from build123d import *

# Parameters (mm, degrees)
BOSS_EXTRUDE1_DEPTH  = 2
SKETCH2_W            = 8
SKETCH2_H            = 8
BOSS_EXTRUDE2_DEPTH  = 2
SKETCH3_W            = 8
SKETCH3_H            = 8
BOSS_EXTRUDE3_DEPTH  = 8
SKETCH4_R            = 3.5
CUT_EXTRUDE1_DEPTH   = 10
CUT_EXTRUDE2_REACH   = 4
SKETCH5_R            = 0.65
CUT_EXTRUDE3_REACH   = 3
SKETCH6_R            = 0.65
SKETCH10_R           = 0.65
BOSS_EXTRUDE6_DEPTH  = 3
SKETCH11_W           = 8
SKETCH11_H           = 2
BOSS_EXTRUDE7_DEPTH  = 8
SKETCH12_R           = 1
CUT_EXTRUDE5_DEPTH   = 8
SKETCH13_W           = 8
SKETCH13_H           = 12
BOSS_EXTRUDE8_DEPTH  = 2
SKETCH14_W           = 8
SKETCH14_H           = 4
BOSS_EXTRUDE9_DEPTH  = 1
BOSS_EXTRUDE10_DEPTH = 2
SKETCH18_R           = 0.65
BOSS_EXTRUDE11_DEPTH = 4
CUT_EXTRUDE6_REACH   = 6
SKETCH19_R           = 0.65
CUT_EXTRUDE7_REACH   = 4
SKETCH20_R           = 1.75


with BuildPart() as part:
    # Sketch1 → Boss-Extrude1 (new body)
    with BuildSketch(Plane(origin=(0, 0, 0), x_dir=(1, 0, 0), z_dir=(0, 1, 0))):
        Polygon((-16, 0), (0, 0), (0, 1), (-8, 1), (-8, 8), (-16, 8), align=None)
    extrude(amount=BOSS_EXTRUDE1_DEPTH)

    # Sketch2 → Boss-Extrude2 (add)
    with BuildSketch(Plane(origin=(0, 2, 0), x_dir=(1, 0, 0), z_dir=(0, 1, 0))):
        with Locations((-12, 4)):
            Rectangle(SKETCH2_W, SKETCH2_H)
    extrude(amount=BOSS_EXTRUDE2_DEPTH)

    # Sketch3 → Boss-Extrude3 (add)
    with BuildSketch(Plane.XZ):
        with Locations((-12, -4)):
            Rectangle(SKETCH3_W, SKETCH3_H)
    extrude(amount=BOSS_EXTRUDE3_DEPTH)

    # Sketch4 → Cut-Extrude1 (cut)
    with BuildSketch(Plane(origin=(0, 4, 0), x_dir=(1, 0, 0), z_dir=(0, 1, 0))):
        with Locations((-12, 4)):
            Circle(SKETCH4_R)
    extrude(amount=-CUT_EXTRUDE1_DEPTH, mode=Mode.SUBTRACT)

    # Sketch5 → Cut-Extrude2 (cut, up to next)
    with BuildSketch(Plane(origin=(0, -6, 0), x_dir=(1, 0, 0), z_dir=(0, 1, 0)), mode=Mode.PRIVATE) as cut_extrude2_sk1:
        with Locations((-13.5, 4)):
            Circle(SKETCH5_R)
    cut_extrude2_tool1 = extrude(cut_extrude2_sk1.sketch, amount=-CUT_EXTRUDE2_REACH, mode=Mode.PRIVATE) & part.part
    add(cut_extrude2_tool1.solids().sort_by_distance((-13.5, -6, -4))[0], mode=Mode.SUBTRACT)
    # Sketch5 → Cut-Extrude2 (cut, up to next)
    with BuildSketch(Plane(origin=(0, -6, 0), x_dir=(1, 0, 0), z_dir=(0, 1, 0)), mode=Mode.PRIVATE) as cut_extrude2_sk2:
        with Locations((-10.5, 4)):
            Circle(SKETCH5_R)
    cut_extrude2_tool2 = extrude(cut_extrude2_sk2.sketch, amount=-CUT_EXTRUDE2_REACH, mode=Mode.PRIVATE) & part.part
    add(cut_extrude2_tool2.solids().sort_by_distance((-10.5, -6, -4))[0], mode=Mode.SUBTRACT)

    # Sketch6 → Cut-Extrude3 (cut, up to next)
    with BuildSketch(Plane(origin=(0, 0, -1), x_dir=(-1, 0, 0), z_dir=(0, 0, -1)), mode=Mode.PRIVATE) as cut_extrude3_sk1:
        with Locations((6.5, 1)):
            Circle(SKETCH6_R)
    cut_extrude3_tool1 = extrude(cut_extrude3_sk1.sketch, amount=-CUT_EXTRUDE3_REACH, mode=Mode.PRIVATE) & part.part
    add(cut_extrude3_tool1.solids().sort_by_distance((-6.5, 1, -1))[0], mode=Mode.SUBTRACT)
    # Sketch6 → Cut-Extrude3 (cut, up to next)
    with BuildSketch(Plane(origin=(0, 0, -1), x_dir=(-1, 0, 0), z_dir=(0, 0, -1)), mode=Mode.PRIVATE) as cut_extrude3_sk2:
        with Locations((4, 1)):
            Circle(SKETCH6_R)
    cut_extrude3_tool2 = extrude(cut_extrude3_sk2.sketch, amount=-CUT_EXTRUDE3_REACH, mode=Mode.PRIVATE) & part.part
    add(cut_extrude3_tool2.solids().sort_by_distance((-4, 1, -1))[0], mode=Mode.SUBTRACT)
    # Sketch6 → Cut-Extrude3 (cut, up to next)
    with BuildSketch(Plane(origin=(0, 0, -1), x_dir=(-1, 0, 0), z_dir=(0, 0, -1)), mode=Mode.PRIVATE) as cut_extrude3_sk3:
        with Locations((1.5, 1)):
            Circle(SKETCH6_R)
    cut_extrude3_tool3 = extrude(cut_extrude3_sk3.sketch, amount=-CUT_EXTRUDE3_REACH, mode=Mode.PRIVATE) & part.part
    add(cut_extrude3_tool3.solids().sort_by_distance((-1.5, 1, -1))[0], mode=Mode.SUBTRACT)

    # Sketch10 → Boss-Extrude6 (add)
    with BuildSketch(Plane.XY):
        Polygon((-8, 2), (-16, 2), (-16, -8), (-8, -8), (-8, 0), (0, 0), (0, 2), align=None)
        with Locations((-1.5, 1)):
            Circle(SKETCH10_R, mode=Mode.SUBTRACT)
        with Locations((-4, 1)):
            Circle(SKETCH10_R, mode=Mode.SUBTRACT)
        with Locations((-6.5, 1)):
            Circle(SKETCH10_R, mode=Mode.SUBTRACT)
    extrude(amount=BOSS_EXTRUDE6_DEPTH)

    # Sketch11 → Boss-Extrude7 (add)
    with BuildSketch(Plane.XZ.offset(8)):
        with Locations((-12, 2)):
            Rectangle(SKETCH11_W, SKETCH11_H)
    extrude(amount=BOSS_EXTRUDE7_DEPTH)

    # Sketch12 → Cut-Extrude5 (cut)
    with BuildSketch(Plane(origin=(0, 0, 1), x_dir=(-1, 0, 0), z_dir=(0, 0, -1))):
        with Locations((12, -12)):
            Circle(SKETCH12_R)
    extrude(amount=-CUT_EXTRUDE5_DEPTH, mode=Mode.SUBTRACT)

    # Sketch13 → Boss-Extrude8 (add)
    with BuildSketch(Plane(origin=(0, 0, -8), x_dir=(-1, 0, 0), z_dir=(0, 0, -1))):
        with Locations((12, -2)):
            Rectangle(SKETCH13_W, SKETCH13_H)
    extrude(amount=BOSS_EXTRUDE8_DEPTH)

    # Sketch14 → Boss-Extrude9 (add)
    with BuildSketch(Plane.XZ):
        with Locations((-4, 1)):
            Rectangle(SKETCH14_W, SKETCH14_H)
    extrude(amount=BOSS_EXTRUDE9_DEPTH)

    # Sketch15 → Boss-Extrude10 (add)
    with BuildSketch(Plane(origin=(0, 2, 0), x_dir=(1, 0, 0), z_dir=(0, 1, 0))):
        Polygon((-8, 0), (-8, 1), (0, 1), (0, -3), (-16, -3), (-16, 0), align=None)
    extrude(amount=BOSS_EXTRUDE10_DEPTH)

    # Sketch18 → Boss-Extrude11 (add)
    with BuildSketch(Plane(origin=(0, 0, -1), x_dir=(-1, 0, 0), z_dir=(0, 0, -1))):
        with Locations((1.5, 1)):
            Circle(SKETCH18_R)
        with Locations((4, 1)):
            Circle(SKETCH18_R)
        with Locations((6.5, 1)):
            Circle(SKETCH18_R)
    extrude(amount=-BOSS_EXTRUDE11_DEPTH)

    # Sketch19 → Cut-Extrude6 (cut, up to next)
    with BuildSketch(Plane(origin=(0, 0, -1), x_dir=(-1, 0, 0), z_dir=(0, 0, -1)), mode=Mode.PRIVATE) as cut_extrude6_sk1:
        with Locations((1.5, 1.5)):
            Circle(SKETCH19_R)
    cut_extrude6_tool1 = extrude(cut_extrude6_sk1.sketch, amount=-CUT_EXTRUDE6_REACH, mode=Mode.PRIVATE) & part.part
    add(cut_extrude6_tool1.solids().sort_by_distance((-1.5, 1.5, -1))[0], mode=Mode.SUBTRACT)
    # Sketch19 → Cut-Extrude6 (cut, up to next)
    with BuildSketch(Plane(origin=(0, 0, -1), x_dir=(-1, 0, 0), z_dir=(0, 0, -1)), mode=Mode.PRIVATE) as cut_extrude6_sk2:
        with Locations((4, 1.5)):
            Circle(SKETCH19_R)
    cut_extrude6_tool2 = extrude(cut_extrude6_sk2.sketch, amount=-CUT_EXTRUDE6_REACH, mode=Mode.PRIVATE) & part.part
    add(cut_extrude6_tool2.solids().sort_by_distance((-4, 1.5, -1))[0], mode=Mode.SUBTRACT)
    # Sketch19 → Cut-Extrude6 (cut, up to next)
    with BuildSketch(Plane(origin=(0, 0, -1), x_dir=(-1, 0, 0), z_dir=(0, 0, -1)), mode=Mode.PRIVATE) as cut_extrude6_sk3:
        with Locations((6.5, 1.5)):
            Circle(SKETCH19_R)
    cut_extrude6_tool3 = extrude(cut_extrude6_sk3.sketch, amount=-CUT_EXTRUDE6_REACH, mode=Mode.PRIVATE) & part.part
    add(cut_extrude6_tool3.solids().sort_by_distance((-6.5, 1.5, -1))[0], mode=Mode.SUBTRACT)

    # Sketch20 → Cut-Extrude7 (cut, up to next)
    with BuildSketch(Plane(origin=(0, 0, 1), x_dir=(-1, 0, 0), z_dir=(0, 0, -1)), mode=Mode.PRIVATE) as cut_extrude7_sk1:
        with Locations((12, -12)):
            Circle(SKETCH20_R)
    cut_extrude7_tool1 = extrude(cut_extrude7_sk1.sketch, amount=-CUT_EXTRUDE7_REACH, mode=Mode.PRIVATE) & part.part
    add(cut_extrude7_tool1.solids().sort_by_distance((-12, -12, 1))[0], mode=Mode.SUBTRACT)


solid = part.part
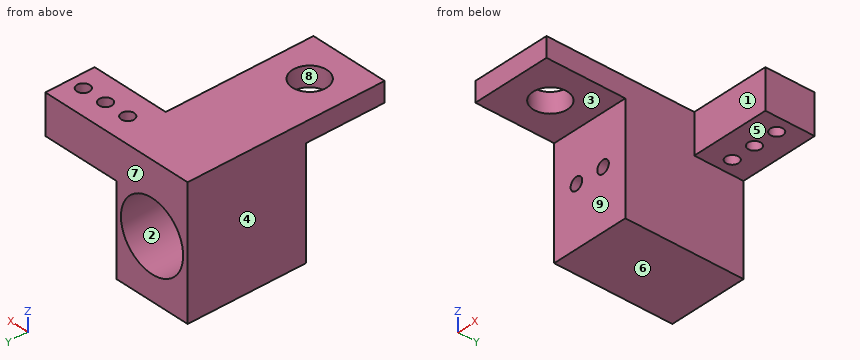
The listing builds one solid part. Answer for the finished solid, in the listing's coordinates (mm). Face numbers are marked on the shaded views. A direction names the side the tool comes from. Round coordinates to 2 decimals unless told otherwise and drop trailing zeros. Write each loop counter-clockwise with the first axis right and the second up, starting at its lowest first coordinate (ties: lowest second). Pieces come first, ordered by that corner, then holes. Notation, with made-up numbers: M -18.75,-21.5 L 34.25,-21.5 A9 ccw 34.25,-9.5 Z; hole C 82.5,26 d6. An arc over 180 degrees is marked long. Write each question's results on one line, items separated by ' | '. Start each with the question number.
Item 1: Find section D-D on y = -12. Write down the section's boundary in (x, z), and give its area (3 significant figures).
Item 2: Straight lines are drawn through the part: probe 1 along Y at (x, z) = (-6.5, 1.25); probe 2 along Z at (x, y) = (-13.5, -6.95); probe 3 along Y at (x, z) = (-5.25, 0.25). For each, find the intervals that lie inside material, in ascending order.
Item 3: The mould has two halves that part along Y. Classify the marked faces 6, 7, 8 and 9: +Y half, -Y half, draft (parallel to the pull), parting line (faces both ways), or undercut.
Item 4: Given pin 1 Ø5 at (x, z) = (-9.5, -4.5) entering from +Y; pin 2 Ø6.5 at (y, z) = (-4, -5) entering from +X; pin 3 Ø1 at (y, z) = (-9, -7) entering from +X; pin 4 Ø3 at (x, z) = (-5, 1) entering from -Y, each flat-ended and moving along its own axis, determine where each tip first touches the part or whether it passes through.
Item 5: Which of the six approach directions +Z, -Z, +X, -X, +Y, -Y give full straight-line access (tool end or side, diameter ignored) to the marked faces 1, 2, 3, 4 and 5?
Item 6: Find section C-C on x = -4. Write down the section's boundary in (y, z).
Item 7: Find section A-A on y = 1.5. Write down the section's boundary in (x, z), and give its area (3 significant figures).
Item 8: Find section B-B on z = -4. Write down the section's boundary in (x, y), and give its area (3 significant figures).
Answer block:
1) outline: M -16,1 L -13.75,1 L -13.75,3 L -16,3 Z; M -10.25,1 L -8,1 L -8,3 L -10.25,3 Z | area: 9.00 mm²
2) probe 1: y = -1 to 0.85, 2.15 to 4 | probe 2: z = -10 to -4.65, -3.35 to 3 | probe 3: y = -1 to 4
3) face 6: draft | face 7: +Y half | face 8: undercut | face 9: -Y half
4) pin 1: stops at y = 4 | pin 2: stops at x = -8 | pin 3: passes through | pin 4: stops at y = -1
5) face 1: +Z, -Z, +X, -Y | face 2: +Y | face 3: -Z, +X, -X, -Y | face 4: +Z, -Z, -X, +Y, -Y | face 5: -Z, +X, +Y, -Y
6) outline: M -1,-1 L 0.85,-1 L 0.85,3 L -1,3 Z; M 2.15,-1 L 4,-1 L 4,3 L 2.15,3 Z
7) outline: M -16,-10 L -8,-10 L -8,-1 L -7.15,-1 L -7.15,3 L -16,3 Z; M -5.85,-1 L -4.65,-1 L -4.65,3 L -5.85,3 Z; M -3.35,-1 L -2.15,-1 L -2.15,3 L -3.35,3 Z; M -0.85,-1 L 0,-1 L 0,3 L -0.85,3 Z; hole C -12,-4 d7 | area: 81.9 mm²
8) outline: M -16,-8 L -14.15,-8 L -14.15,-6 L -15.5,-6 L -15.5,4 L -16,4 Z; M -12.85,-8 L -11.15,-8 L -11.15,-6 L -12.85,-6 Z; M -9.85,-8 L -8,-8 L -8,4 L -8.5,4 L -8.5,-6 L -9.85,-6 Z | area: 20.8 mm²
